Design review of the part built by this model. Coordinates are the model's own, in mm. Face numbers are marked on the shaded views. A direction names the side the tool comes from. Coordinates: 2 decimals unless noted, no trailing zeros. Loops run counter-clockwise (first coordinate to the right, second up) from the corner with the lowest first, then second, coordinate; pieces in that order, holes last. Notation, with made-up numbers: (-18.75, 35) -> (8.25, 35) arc R21 cw to (8.25, 72) -> close; hole circle Ø1 at (36, 18.5). An arc over 180 degrees is marked (long way). Answer in a Markdown table with one row per item.
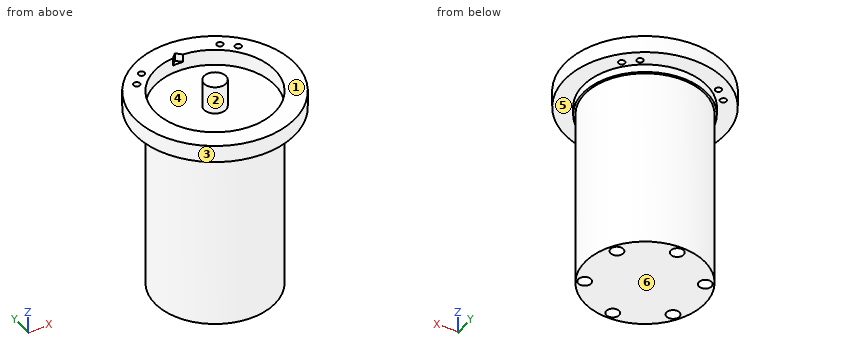
```python
from build123d import *

# Parameters (mm, degrees)
SKETCH_2_R          = 15.5
EXTRUDE_1_DEPTH     = 2
SKETCH_3_R          = 15
EXTRUDE_2_DEPTH     = 45
SKETCH_4_R          = 20
EXTRUDE_3_DEPTH     = 4.3
SKETCH_5_R          = 15
CUT_EXTRUDE_2_DEPTH = 4
SKETCH_6_R          = 2.75
EXTRUDE_4_DEPTH     = 7
SKETCH_7_R          = 0.8
CUT_EXTRUDE_3_DEPTH = 7
CUT_EXTRUDE_4_DEPTH = 2
SKETCH_10_R         = 1.6
CUT_EXTRUDE_5_DEPTH = 10


with BuildPart() as part:
    # 草图2 → 凸台-拉伸1 (new body)
    with BuildSketch(Plane.XY):
        Circle(SKETCH_2_R)
    extrude(amount=EXTRUDE_1_DEPTH)

    # 草图3 → 凸台-拉伸2 (add)
    with BuildSketch(Plane(origin=(0, 0, 0), x_dir=(-1, 0, 0), z_dir=(0, 0, -1))):
        with Locations(Location((0, 0, 0), (0, 0, 180))):
            Circle(SKETCH_3_R)
    extrude(amount=EXTRUDE_2_DEPTH)

    # 草图4 → 凸台-拉伸3 (add)
    with BuildSketch(Plane.XY.offset(2)):
        with Locations(Location((0, 0, 0), (0, 0, 180))):
            Circle(SKETCH_4_R)
    extrude(amount=EXTRUDE_3_DEPTH)

    # 草图5 → 切除-拉伸2 (cut)
    with BuildSketch(Plane.XY.offset(6.3)):
        Circle(SKETCH_5_R)
    extrude(amount=-CUT_EXTRUDE_2_DEPTH, mode=Mode.SUBTRACT)

    # 草图6 → 凸台-拉伸4 (add)
    with BuildSketch(Plane.XY.offset(2.3)):
        Circle(SKETCH_6_R)
    extrude(amount=EXTRUDE_4_DEPTH)

    # 草图7 → 切除-拉伸3 (cut)
    with BuildSketch(Plane.XY.offset(6.3)):
        with Locations((-10, 13.809507594)):
            Circle(SKETCH_7_R)
        with Locations((10, 13.809507594)):
            Circle(SKETCH_7_R)
        with Locations((-12.95, 11.090536506)):
            Circle(SKETCH_7_R)
        with Locations((12.95, 11.090536506)):
            Circle(SKETCH_7_R)
    extrude(amount=-CUT_EXTRUDE_3_DEPTH, mode=Mode.SUBTRACT)

    # 草图9 → 切除-拉伸4 (cut)
    with BuildSketch(Plane.XY.offset(6.3)):
        Polygon((-2.828427125, 13.378), (0, 16.206427125), (2.828427125, 13.378), (0, 10.549572875), align=None)
    extrude(amount=-CUT_EXTRUDE_4_DEPTH, mode=Mode.SUBTRACT)

    # 草图10 → 切除-拉伸5 (cut)
    with BuildSketch(Plane(origin=(0, 0, -45), x_dir=(-1, 0, 0), z_dir=(0, 0, -1))):
        with Locations((11.258330249, 6.5)):
            Circle(SKETCH_10_R)
        with Locations((0, 13)):
            Circle(SKETCH_10_R)
        with Locations((11.258330249, -6.5)):
            Circle(SKETCH_10_R)
        with Locations((0, -13)):
            Circle(SKETCH_10_R)
        with Locations((-11.258330249, -6.5)):
            Circle(SKETCH_10_R)
        with Locations((-11.258330249, 6.5)):
            Circle(SKETCH_10_R)
    extrude(amount=-CUT_EXTRUDE_5_DEPTH, mode=Mode.SUBTRACT)


solid = part.part
```
(1) Take a section at D-D on y = -13. Give the boundary of the cut face in (x, z).
Evaluation:
| item | result |
|---|---|
| outline | (-15.2, 2) -> (-8.44, 2) -> (-8.44, 0) -> (-7.48, 0) -> (-7.48, -45) -> (-1.6, -45) -> (-1.6, -35) -> (1.6, -35) -> (1.6, -45) -> (7.48, -45) -> (7.48, 0) -> (8.44, 0) -> (8.44, 2) -> (15.2, 2) -> (15.2, 6.3) -> (7.48, 6.3) -> (7.48, 2.3) -> (-7.48, 2.3) -> (-7.48, 6.3) -> (-15.2, 6.3) -> close |
(2) Draft analysis for pull direction X (two halves, no side actions). For the marked faces 1, 2, 3 and 4, state which applies: pulls with the +X half, pulls with the -X half, needs draft (parallel to the pull), parting line crosses it, or undercut.
Evaluation:
| item | result |
|---|---|
| face 1 | needs draft |
| face 2 | undercut |
| face 3 | parting line crosses it |
| face 4 | undercut |
(3) For pin 1 (12 mm diameter, centred on x = 4, y = 14, fed in from +Z); pin 2 (3 mm diameter, centred on x = 0, y = -13, fed in from +Z); pin 3 (1 mm diameter, centred on x = -12, y = 13, fed in from -Z), all flat-tipped, find the tip position at first contact; note any pin that passes through.
Evaluation:
| item | result |
|---|---|
| pin 1 | stops at z = 6.3 |
| pin 2 | stops at z = 2.3 |
| pin 3 | stops at z = 2 |
(4) Take a section at A-A on y = 0. Give the boundary of the cut face in (x, z), and give its area (3 significant figures).
Evaluation:
| item | result |
|---|---|
| outline | (-20, 2) -> (-15.5, 2) -> (-15.5, 0) -> (-15, 0) -> (-15, -45) -> (15, -45) -> (15, 0) -> (15.5, 0) -> (15.5, 2) -> (20, 2) -> (20, 6.3) -> (15, 6.3) -> (15, 2.3) -> (2.75, 2.3) -> (2.75, 9.3) -> (-2.75, 9.3) -> (-2.75, 2.3) -> (-15, 2.3) -> (-15, 6.3) -> (-20, 6.3) -> close |
| area | 1,500 mm² |
(5) Take a section at C-C on x = -4.5. Give the boundary of the cut face in (y, z), and give its area (3 significant figures).
Evaluation:
| item | result |
|---|---|
| outline | (-19.49, 2) -> (-14.83, 2) -> (-14.83, 0) -> (-14.31, 0) -> (-14.31, -45) -> (14.31, -45) -> (14.31, 0) -> (14.83, 0) -> (14.83, 2) -> (19.49, 2) -> (19.49, 6.3) -> (14.31, 6.3) -> (14.31, 2.3) -> (-14.31, 2.3) -> (-14.31, 6.3) -> (-19.49, 6.3) -> close |
| area | 1,400 mm² |
(6) Tool access review of the marked faces 5 and 6: name each direction out of +Z, -Z, +X, -X, +Y, -Y from which nothing blocks a thin tool from reaching the whole face with its end or side.
Evaluation:
| item | result |
|---|---|
| face 5 | -Z |
| face 6 | -Z, +X, -X, +Y, -Y |
(7) Take a section at B-B on z = -13. Give the boundary of the cut face in (x, y).
Evaluation:
| item | result |
|---|---|
| outline | circle Ø30 at (0, 0) |
(8) To check wall thickness, follow probe 1 along Y at (x, z) = (0, -43); probe 2 along X at (y, z) = (-6, -37); probe 3 along Z at (x, y) = (-12, -10.5). State the ranges of each line that lie inside material, in increasing order.
Evaluation:
| item | result |
|---|---|
| probe 1 | y = -15 to -14.6, -11.4 to 11.4, 14.6 to 15 |
| probe 2 | x = -13.75 to -12.78, -9.74 to 9.74, 12.78 to 13.75 |
| probe 3 | z = 2 to 6.3 |
